Check sheet for the modelled part. Datum: model origin and axes. Units: mm. Coordinates: 2 decimals unless noted, no trailing zeros. Loops run counter-clockwise (first coordinate to the right, second up) from the corner with the lowest first, then second, coordinate; pieces in that order, holes last. Notation, with made-up numbers: (76.25, -38.5) -> (103.25, -38.5) arc R27 ccw to (103.25, -4.5) -> close; hole circle Ø8 at (8.5, 27). An arc over 180 degrees is marked (long way). Use CSV: the item, a comma, the result in double quotes. Start each with the question number.
1. Sectioned sample at A-A, the plane z = -60. Record the cut outline in (x, y), and give its area (3 significant figures).
2. Gauge pin test, flat ends, axial feed: pin 1 (7.5 mm diameter, centred on x = 0, z = 29, fed in from +Y); pin 2 (3.5 mm diameter, centred on x = 10, z = -7, fed in from -Y). Record the tip position at first contact, or that the pin passes through.
3. Thickness scan on L1, parallel to X at y = 6.25, z = -7; L2, parallel to Z at x = 0, y = 4; L3, parallel to Z at x = 10, y = 3.25. Record the ranges inside material, lowest first.
4. Sectioned sample at D-D, the plane z = -37. Record the cut outline in (x, y), and give its area (3 significant figures).
5. Sectioned sample at C-C, the plane x = -10. Record the cut outline in (y, z).
6. Sectioned sample at B-B, the plane y = 7. Record the cut outline in (x, z), and give its area (3 significant figures).
Autodesk Inventor part; units mm, degrees
ref_plane "YZ Plane" through (0, 0, 0) normal (1, 0, 0) x (0, 1, 0)
ref_plane "XZ Plane" through (0, 0, 0) normal (0, 1, 0) x (-1, 0, 0)
ref_plane "XY Plane" through (0, 0, 0) normal (0, 0, 1) x (1, 0, 0)
sketch "Sketch1" plane through (0, 0, 0) normal (0, 1, 0) x (-1, 0, 0)
  line L0 (-15, -65) -> (15, -65)
  line L1 (15, -65) -> (15, 65)
  line L2 (15, 65) -> (-15, 65)
  line L3 (-15, 65) -> (-15, -65)
  line L4 (-15, -65) -> (15, 65) construction
  line L5 (15, -65) -> (-15, 65) construction
  point P0 (0, 0)
  dimension "d0" = 30
  dimension "d1" = 130
extrude "Extrusion1" add sketch "Sketch1" along normal blind 10
sketch "Sketch2" plane through (0, 10, 0) normal (0, 1, 0) x (1, 0, 0)
  line L0 (15, 65) -> (-15, 65)
  point P0 (0, 0)
  point P1 (0, -29)
  point P2 (0, -54)
  dimension "d4" = 94
  dimension "d5" = 25
hole "Hole1" at (0, 10, 29) at (0, 10, 54) direction (0, -1, 0) diameter 6.647 depth 22.2 tip angle 118
sketch "Sketch3" plane through (0, 0, 0) normal (0, -1, 0) x (1, 0, 0)
  line L0 (15, -65) -> (-15, -65)
  line L1 (-15, -65) -> (-15, 65)
  point P0 (0, 0)
  point P1 (0, -60)
  dimension "d13" = 5
  dimension "d14" = 15
hole "Hole2" at (0, 0, -60) direction (0, 1, 0) diameter 4.917 end through all
sketch "Sketch4" plane through (0, 0, 0) normal (0, -1, 0) x (1, 0, 0)
  line L0 (10, -37) -> (-10, -37) construction
  line L1 (-10, -37) -> (-10, -7) construction
  line L2 (-10, -7) -> (10, -7) construction
  line L3 (10, -7) -> (10, -37) construction
  line L4 (15, -65) -> (-15, -65) construction
  line L5 (15, 65) -> (15, -65) construction
  point P0 (0, 0)
  dimension "d22" = 20
  dimension "d23" = 30
  dimension "d24" = 28
  dimension "d25" = 5
hole "Hole3" at (10, 0, -37) at (-10, 0, -37) at (-10, 0, -7) at (10, 0, -7) direction (0, 1, 0) diameter 4.134 end through all
chamfer "Chamfer1" distance 2 angle 45 8 edges at (15, 5, -65) (-15, 5, -65) (15, 5, 65) (15, 0, 0) (0, 0, -65) (-15, 0, 0) (0, 0, 65) (-15, 5, 65)
properties part number "Horizontal_support" material "Stainless Steel"
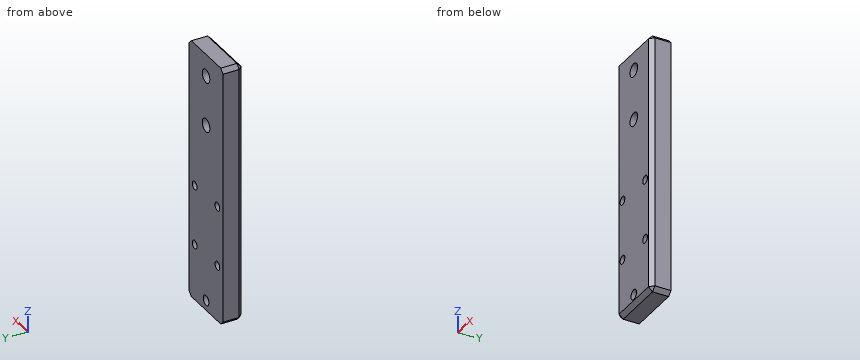
Completed:
1,outline,"(-15, 2) -> (-13, 0) -> (-2.46, 0) -> (-2.46, 10) -> (-15, 10) -> close; (2.46, 0) -> (13, 0) -> (15, 2) -> (15, 10) -> (2.46, 10) -> close"
1,area,"247 mm²"
2,pin 1,"y = 10"
2,pin 2,"through"
3,L1,"-15 to -12.07, -7.93 to 7.93, 12.07 to 15"
3,L2,"-65 to -62.46, -57.54 to 25.68, 32.32 to 50.68, 57.32 to 65"
3,L3,"-65 to -39.07, -34.93 to -9.07, -4.93 to 65"
4,outline,"(-15, 2) -> (-13, 0) -> (-12.07, 0) -> (-12.07, 10) -> (-15, 10) -> close; (-7.93, 0) -> (7.93, 0) -> (7.93, 10) -> (-7.93, 10) -> close; (12.07, 0) -> (13, 0) -> (15, 2) -> (15, 10) -> (12.07, 10) -> close"
4,area,"213 mm²"
5,outline,"(0, -63) -> (2, -65) -> (10, -65) -> (10, -39.07) -> (0, -39.07) -> close; (0, -34.93) -> (10, -34.93) -> (10, -9.07) -> (0, -9.07) -> close; (0, -4.93) -> (10, -4.93) -> (10, 65) -> (2, 65) -> (0, 63) -> close"
6,outline,"(-15, -63) -> (-13, -65) -> (13, -65) -> (15, -63) -> (15, 63) -> (13, 65) -> (-13, 65) -> (-15, 63) -> close; hole circle Ø4.13 at (-10, -37); hole circle Ø4.13 at (-10, -7); hole circle Ø6.65 at (0, 29); hole circle Ø6.65 at (0, 54); hole circle Ø4.92 at (0, -60); hole circle Ø4.13 at (10, -37); hole circle Ø4.13 at (10, -7)"
6,area,"3,750 mm²"
